The listing builds one solid part. Answer for the finished solid, in the listing's coordinates (mm). Face numbers are marked on the shaded views. A direction names the side the tool comes from. Give positions to 0.01 mm unless a question says otherwise; leave off trailing zeros. Order: outer loops, then holes, each group sorted by start corner. A loop starts at its lowest first (then second) coordinate and runs counter-clockwise, first axis right, second up. Notation, with made-up numbers: (-8.75, -31.5) - (41.25, -31.5) arc R17 cw to (41.25, -16.5) - close; hole circle Ø5 at (6, 43). An arc over 180 degrees is marked (long way). Answer in a Markdown table with one row per item.
Autodesk Inventor part; units mm, degrees
ref_plane "YZ Plane" through (0, 0, 0) normal (1, 0, 0) x (0, 1, 0)
ref_plane "XZ Plane" through (0, 0, 0) normal (0, 1, 0) x (-1, 0, 0)
ref_plane "XY Plane" through (0, 0, 0) normal (0, 0, 1) x (1, 0, 0)
sketch "Skizze1" plane through (0, 0, 0) normal (0, 1, 0) x (-1, 0, 0)
  circle A0 centre (0, 0) radius 2.5
  dimension "d0" = 5
extrude "Höhe" add sketch "Skizze1" along normal blind 8
fillet "Radius_Kopf" radius 2.5 1 edges at (2.5, 8, 0)
sketch "Skizze2" plane through (0, 0, 0) normal (0, -1, 0) x (1, 0, 0)
  arc A0 (-1.6583, 2.5) -> (1.6583, 2.5) centre (0, 0) ccw
  line L0 (-1.6583, 2.5) -> (1.6583, 2.5)
  circle A1 centre (0, 0) radius 2.5
  dimension "d4" = 6
extrude "Kante" add sketch "Skizze2" along normal blind 1 contours A1 | L0 A0
sketch "Skizze3" plane through (0, -1, 0) normal (0, -1, 0) x (1, 0, 0)
  circle A0 centre (0, 0) radius 2.5 construction
  line L0 (0, 2.5) -> (0, -3) construction
  arc A1 (-1.6583, 2.5) -> (1.6583, 2.5) centre (0, 0) ccw construction
  line L1 (-2.5, 0) -> (2.5, 0) construction
  line L2 (-0.25, 1.52) -> (0.25, 1.52)
  line L3 (0.25, 1.52) -> (0.25, 1.02)
  line L4 (0.25, 1.02) -> (-0.25, 1.02)
  line L5 (-0.25, 1.02) -> (-0.25, 1.52)
  line L6 (-0.25, 1.27) -> (0.25, 1.27) construction
  line L7 (-0.25, -1.52) -> (0.25, -1.52)
  line L8 (0.25, -1.52) -> (0.25, -1.02)
  line L9 (0.25, -1.02) -> (-0.25, -1.02)
  line L10 (-0.25, -1.02) -> (-0.25, -1.52)
  point P0 (0, 1.27)
  point P1 (0, -1.27)
  dimension "d7" = 2.54
  dimension "d8" = 0.5
  dimension "d9" = 0.5
extrude "Pin" add sketch "Skizze3" along normal blind 5
properties part number "LED_5mm_Gelb"
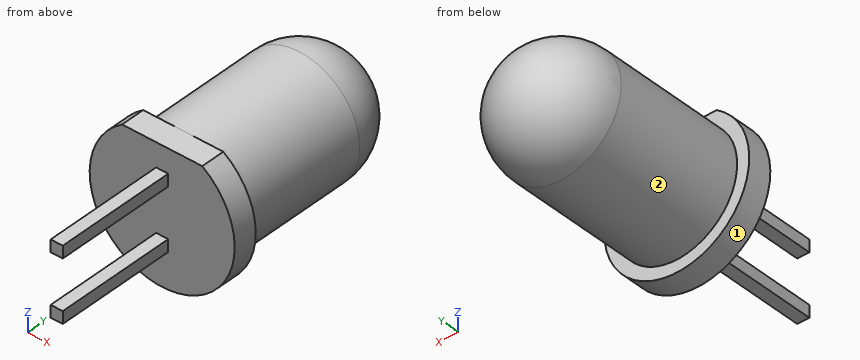
Item 1: Each of these flat-tipped pins is pushed along its axis until it touches: P1, Ø0.6, axis at x = 0, y = -4.5, coming from the -Z side; P2, Ø0.6, axis at y = -2.5, z = -1.5, coming from the +X side; P3, Ø1, axis at x = 2, y = 2, coming from the -Z side. Where does it stop, or does it pass through?
Answer block:
| item | result |
|---|---|
| P1 | z = -1.52 |
| P2 | x = 0.25 |
| P3 | z = -2 |
Item 2: Which of the six approach directions +Z, -Z, +X, -X, +Y, -Y give full straight-line access (tool end or side, diameter ignored) to the marked faces 1 and 2?
Answer block:
| item | result |
|---|---|
| face 1 | +Y, -Y |
| face 2 | +Y |
Item 3: Consider line 1 (Z direction, x = 0.2, y = -2.5); line 2 (Y direction, x = 1.25, z = 0.1); line 3 (Y direction, x = 0.6, z = -0.8). Determine where each line is inside the solid, lowest interval first.
Answer block:
| item | result |
|---|---|
| line 1 | -1.52 to -1.02, 1.02 to 1.52 |
| line 2 | -1 to 7.66 |
| line 3 | -1 to 7.79 |
Item 4: Find section D-D on y = 4.5. Write down the section's boundary in (x, z), then the cut area to 3 significant figures.
Answer block:
| item | result |
|---|---|
| outline | circle Ø5 at (0, 0) |
| area | 19.6 mm² |
Item 5: Find section C-C on x = 2.25. Write down the section's boundary in (y, z), then the cut area to 3 significant figures.
Answer block:
| item | result |
|---|---|
| outline | (-1, -1.98) - (0, -1.98) - (0, -1.09) - (5.5, -1.09) arc R1.09 ccw to (5.5, 1.09) - (0, 1.09) - (0, 1.98) - (-1, 1.98) - close |
| area | 17.8 mm² |
Item 6: Find section A-A on y = -3.5. Write down the section's boundary in (x, z), then the cut area to 3 significant figures.
Answer block:
| item | result |
|---|---|
| outline | (-0.25, -1.52) - (0.25, -1.52) - (0.25, -1.02) - (-0.25, -1.02) - close; (-0.25, 1.02) - (0.25, 1.02) - (0.25, 1.52) - (-0.25, 1.52) - close |
| area | 0.500 mm² |
Item 7: Find section B-B on z = 0. Write down the section's boundary in (x, y).
Answer block:
| item | result |
|---|---|
| outline | (-3, -1) - (3, -1) - (3, 0) - (2.5, 0) - (2.5, 5.5) arc R2.5 ccw to (-2.5, 5.5) - (-2.5, 0) - (-3, 0) - close |
